```python
from build123d import *

# Parameters (mm, degrees)
F0_R     = 20
F0_R_2   = 18.589258
F0_R_3   = 68.575509
F1_DEPTH = 25
F0_R_4   = 5
F2_DEPTH = 5


with BuildPart() as f1:
    # F0 (on Right) → F1 (new body)
    with BuildSketch(Plane.YZ):
        with BuildLine():
            Line((-298.589258, 0), (0, 0))
            Line((0, 0), (0, 892.051685))
            ThreePointArc((0, 892.051685), (-54.630274, 1257.867666), (-213.75398, 1591.762028))
            ThreePointArc((-213.75398, 1591.762028), (-665.110466, 1751.764013), (-950, 1366.846793))
            Line((-950, 1366.846793), (-950, 1253.181696))
            Line((-950, 1253.181696), (-950, 1250))
            Line((-950, 1250), (-850, 1250))
            Line((-850, 1250), (-558.699328, 1250))
            ThreePointArc((-558.699328, 1250), (-374.773734, 1173.815524), (-298.589258, 989.88993))
            Line((-298.589258, 989.88993), (-298.589258, 0))
        make_face()
        with Locations((-250.612468, 51.013041)):
            Circle(F0_R, mode=Mode.SUBTRACT)
        with Locations((-250, 251.013041)):
            Circle(F0_R, mode=Mode.SUBTRACT)
        with Locations((-248.589258, 451.013041)):
            Circle(F0_R, mode=Mode.SUBTRACT)
        with Locations((-250, 651.013041)):
            Circle(F0_R_2, mode=Mode.SUBTRACT)
        with Locations((-250, 851.013041)):
            Circle(F0_R, mode=Mode.SUBTRACT)
        with Locations((-900, 1300)):
            Circle(F0_R, mode=Mode.SUBTRACT)
        with Locations((-851.884544, 1470.595476)):
            Circle(F0_R, mode=Mode.SUBTRACT)
        with Locations((-721.809268, 1591.004512)):
            Circle(F0_R, mode=Mode.SUBTRACT)
        with Locations((-575, 1437.5)):
            Circle(F0_R_3, mode=Mode.SUBTRACT)
        with Locations((-548.01309, 1625.829824)):
            Circle(F0_R, mode=Mode.SUBTRACT)
        with Locations((-250, 1051.013041)):
            Circle(F0_R, mode=Mode.SUBTRACT)
        with Locations((-250, 1250)):
            Circle(F0_R, mode=Mode.SUBTRACT)
        with Locations((-271.458319, 1425.947305)):
            Circle(F0_R, mode=Mode.SUBTRACT)
        with Locations((-381.587799, 1564.83363)):
            Circle(F0_R, mode=Mode.SUBTRACT)
    extrude(amount=F1_DEPTH)

    # F0 (on Right) → F2 (join)
    with BuildSketch(Plane.YZ):
        with Locations((-250.612468, 51.013041)):
            Circle(F0_R)
        with Locations((-250.612468, 51.013041)):
            Circle(F0_R_4, mode=Mode.SUBTRACT)
        with Locations((-250, 251.013041)):
            Circle(F0_R)
        with Locations((-250, 251.013041)):
            Circle(F0_R_4, mode=Mode.SUBTRACT)
        with Locations((-248.589258, 451.013041)):
            Circle(F0_R)
        with Locations((-248.589258, 451.013041)):
            Circle(F0_R_4, mode=Mode.SUBTRACT)
        with Locations((-250, 651.013041)):
            Circle(F0_R_2)
        with Locations((-250, 651.013041)):
            Circle(F0_R_4, mode=Mode.SUBTRACT)
        with Locations((-250, 851.013041)):
            Circle(F0_R)
        with Locations((-250, 851.013041)):
            Circle(F0_R_4, mode=Mode.SUBTRACT)
        with Locations((-250, 1051.013041)):
            Circle(F0_R)
        with Locations((-250, 1051.013041)):
            Circle(F0_R_4, mode=Mode.SUBTRACT)
        with Locations((-250, 1250)):
            Circle(F0_R)
        with Locations((-250, 1250)):
            Circle(F0_R_4, mode=Mode.SUBTRACT)
        with Locations((-271.458319, 1425.947305)):
            Circle(F0_R)
        with Locations((-271.458319, 1425.947305)):
            Circle(F0_R_4, mode=Mode.SUBTRACT)
        with Locations((-381.587799, 1564.83363)):
            Circle(F0_R)
        with Locations((-381.587799, 1564.83363)):
            Circle(F0_R_4, mode=Mode.SUBTRACT)
        with Locations((-548.01309, 1625.829824)):
            Circle(F0_R)
        with Locations((-548.01309, 1625.829824)):
            Circle(F0_R_4, mode=Mode.SUBTRACT)
        with Locations((-721.809268, 1591.004512)):
            Circle(F0_R)
        with Locations((-721.809268, 1591.004512)):
            Circle(F0_R_4, mode=Mode.SUBTRACT)
        with Locations((-851.884544, 1470.595476)):
            Circle(F0_R)
        with Locations((-851.884544, 1470.595476)):
            Circle(F0_R_4, mode=Mode.SUBTRACT)
        with Locations((-900, 1300)):
            Circle(F0_R)
        with Locations((-900, 1300)):
            Circle(F0_R_4, mode=Mode.SUBTRACT)
    extrude(amount=F2_DEPTH)


solid = f1.part
```
Can you work these out from the model? Positions are in its coordinate system, mm. A direction names the side the tool comes from. Coordinates: 2 decimals unless noted, no trailing zeros. Loops run counter-clockwise (first coordinate to the right, second up) from the corner with the lowest first, then second, coordinate; pieces in that order, holes last.
Item 1: I'm going to push flat-ended pins straight in: pin 1 (6 mm diameter, centred on y = -250, z = 1250, fed in from -X); pin 2 (12 mm diameter, centred on y = -246, z = 248, fed in from +X); pin 3 (8 mm diameter, centred on x = 8, y = -663, fed in from +Z); pin 4 (1 mm diameter, centred on x = 15.5, y = -318.5, fed in from +Z). Where does each tip first touch, or does it pass through?
Answers below:
pin 1: passes through
pin 2: stops at x = 5
pin 3: stops at z = 1753.58
pin 4: stops at z = 1698.16
Item 2: Suppose I cut it at C-C (y = -77.5). Please give me the cut outline in (x, z), then the cut area to 3 significant figures.
Answers below:
outline: (0, 0) - (25, 0) - (25, 1325.72) - (0, 1325.72) - close
area: 33,100 mm2
Item 3: Suppose I cut it at A-A (y = -623.5). Please give me the cut outline in (x, z), then the cut area to 3 significant figures.
Answers below:
outline: (0, 1250) - (25, 1250) - (25, 1389.02) - (0, 1389.02) - close; (0, 1485.98) - (25, 1485.98) - (25, 1762.09) - (0, 1762.09) - close
area: 10,400 mm2
Item 4: Suppose I cut it at B-B (z = 707.5). Please give me the cut outline in (x, y).
Answers below:
outline: (0, -298.59) - (25, -298.59) - (25, 0) - (0, 0) - close
Item 5: Please list where these lines run through material, in increasing order: L1, parallel to Y at x = 1, z = 374; L2, parallel to Y at x = 3, z = 908.5; L3, parallel to Z at x = 15.25, y = -553.5.
Answers below:
L1: y = -298.59 to 0
L2: y = -298.59 to -0.11
L3: z = 1249.95 to 1372.38, 1502.62 to 1606.6, 1645.06 to 1769.28
Item 6: Which directions (+Z, -Z, +X, -X, +Y, -Y) give clear straight access to the entire face, cutting with the end or side of a thin tool? Please do faces 4 (the face through (14.86, -711.06, 1607.87)), 5 (the face through (0, -271, 1094)).
Answers below:
face 4: +X
face 5: +Z, -Z, -X, +Y, -Y
Item 7: If we mould it in two halves opening along Z, with no side actions, what happens to faces 1 (the face through (14.86, -252.6, 1269.83)), 2 (the face through (12.32, -53.12, 1252.89)), 3 (the face through (12.32, -376.81, 1175.83))? For each: released by +Z, released by -Z, zero draft, split by the parting line, or undercut.
Answers below:
face 1: undercut
face 2: released by +Z
face 3: released by -Z
